Print and shaded views of the part. All mm, measured from the part's lowest x, y and z. Round coordinates to 2 decimals unless told otherwise and drop trailing zeros. Order: outer loops, then holes, each group sorted by start corner. A loop starts at its lowest first (then second) coordinate and runs counter-clockwise, first axis right, second up. Notation, with made-up numbers: M 15.5,47.25 L 47.5,47.25 A25 cw 47.5,75.25 Z; hole C 63.5,-27.75 d8. An arc over 180 degrees is marked long. Write each question's results on one line, items separated by ' | '. Start each with the question number.
1. Probe L1, parallel to Z at x = 31.75, y = 8.5; L2, parallel to X at y = 10.5, z = 30.5; L3, parallel to Z at x = 28.5, y = 1.25. List the from-to ranges inside material, lowest first. Write a range as [from, to].
2. Drop flat-ended pins along their axis: pin 1 Ø2 at (x, y) = (11.5, 4.5) entering from +Z; pin 2 Ø5 at (y, z) = (7, 23.5) entering from -X. Give the stop position or say it passes through.
3. Two-plate mould, pull along Z, no slides. Class the marked faces 1, 2, 3 and 4: +Z half, -Z half, draft (parallel to the pull), parting line (faces both ways), or undercut.
4. Band-saw the part on A-A, the plane z = 31.75. List the corners of the cut face in (x, y), then the cut area to 3 significant figures.
5. Band-saw the part on B-B, the plane y = 11. List the corners of the cut face in (x, z).
6. Band-saw the part on D-D, the plane x = 7.5. List the corners of the cut face in (y, z).
7. Band-saw the part on C-C, the plane x = 31.75. List the corners of the cut face in (y, z).
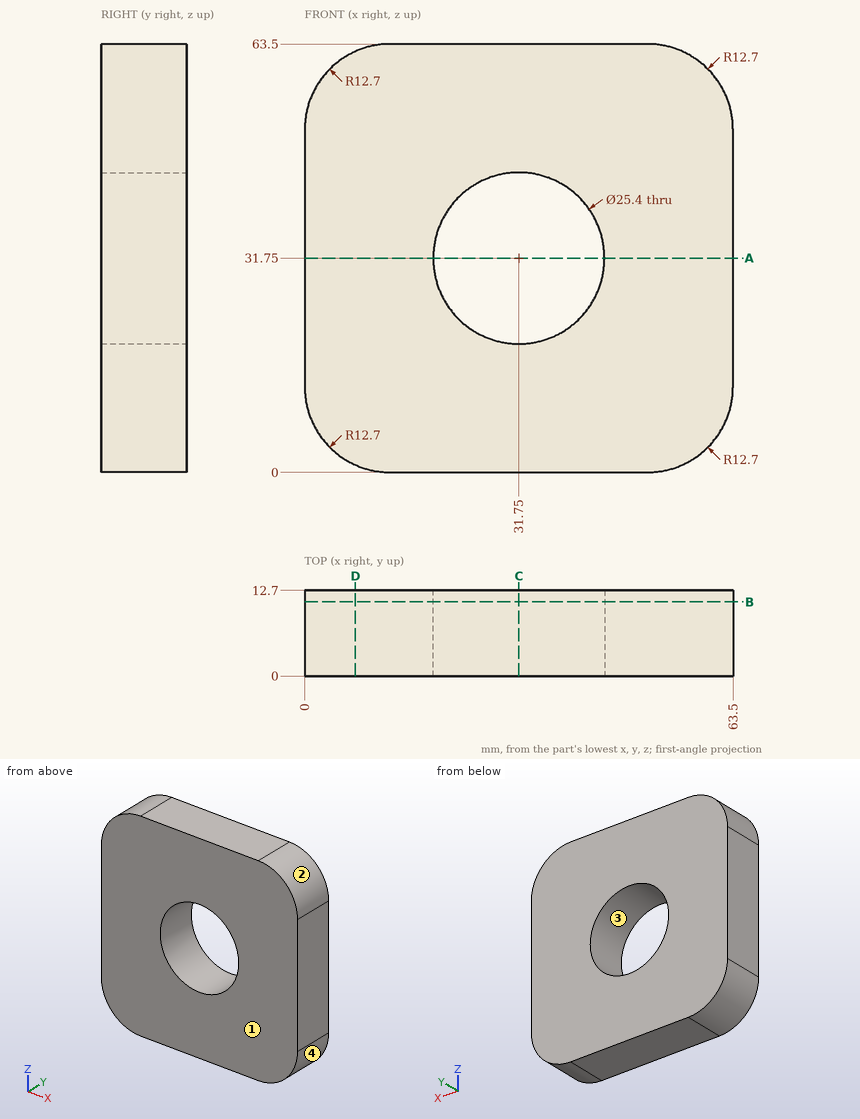
Solution:
1) L1: [0, 19.05], [44.45, 63.5] | L2: [0, 19.11], [44.39, 63.5] | L3: [0, 19.47], [44.03, 63.5]
2) pin 1: z = 63.5 | pin 2: x = 0
3) face 1: draft | face 2: +Z half | face 3: undercut | face 4: -Z half
4) outline: M 0,0 L 19.05,0 L 19.05,12.7 L 0,12.7 Z; M 44.45,0 L 63.5,0 L 63.5,12.7 L 44.45,12.7 Z | area: 484 mm^2
5) outline: M 0,12.7 A12.7 ccw 12.7,0 L 50.8,0 A12.7 ccw 63.5,12.7 L 63.5,50.8 A12.7 ccw 50.8,63.5 L 12.7,63.5 A12.7 ccw 0,50.8 Z; hole C 31.75,31.75 d25.4
6) outline: M 0,1.11 L 12.7,1.11 L 12.7,62.39 L 0,62.39 Z
7) outline: M 0,0 L 12.7,0 L 12.7,19.05 L 0,19.05 Z; M 0,44.45 L 12.7,44.45 L 12.7,63.5 L 0,63.5 Z
